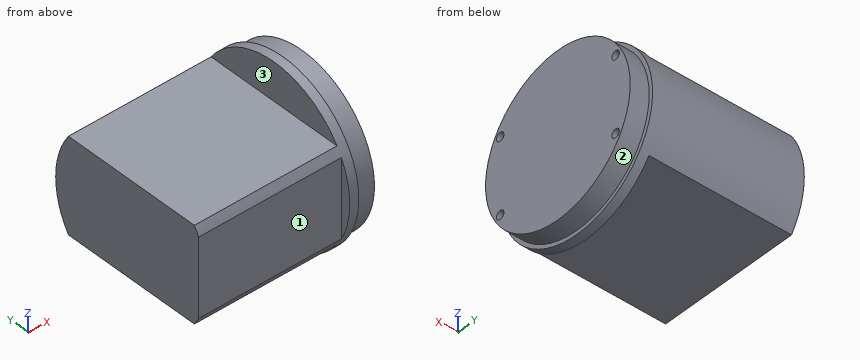
from build123d import *

# Parameters (mm, degrees)
F0_R     = 28.575
F0_R_2   = 27.2923
F1_DEPTH = 57.15
F2_DEPTH = 6.35
F4_DEPTH = 47.752
F5_R     = 1.4224
F6_DEPTH = 9.652


with BuildPart() as f1:
    # F0 (on Right) → F1 (new body)
    with BuildSketch(Plane.YZ):
        Circle(F0_R)
        Circle(F0_R_2, mode=Mode.SUBTRACT)
        Circle(F0_R_2)
    extrude(amount=-F1_DEPTH)

    # F0 (on Right) → F2 (cut)
    with BuildSketch(Plane.YZ):
        Circle(F0_R)
        Circle(F0_R_2, mode=Mode.SUBTRACT)
    extrude(amount=-F2_DEPTH, mode=Mode.SUBTRACT)

    # F3 (on face) → F4 (cut)
    with BuildSketch(Plane(origin=(-57.15, 0, 0), x_dir=(0, -1, 0), z_dir=(-1, 0, 0))):
        with BuildLine():
            ThreePointArc((-23.759524406, -15.875), (0, -28.575), (23.759524406, -15.875))
            Line((23.759524406, -15.875), (-23.759524406, -15.875))
        make_face()
        with BuildLine():
            Line((25.4, 13.0908603613), (25.4, -13.0908603613))
            ThreePointArc((25.4, -13.0908603613), (27.7699083992, -6.7351920908), (28.575, 0))
            ThreePointArc((28.575, 0), (27.7699083992, 6.7351920908), (25.4, 13.0908603613))
        make_face()
        with BuildLine():
            Line((-23.759524406, 15.875), (23.759524406, 15.875))
            ThreePointArc((23.759524406, 15.875), (0, 28.575), (-23.759524406, 15.875))
        make_face()
    extrude(amount=-F4_DEPTH, mode=Mode.SUBTRACT)

    # F5 (on face) → F6 (cut)
    with BuildSketch(Plane.YZ):
        with Locations((-21.7678, 12.573)):
            Circle(F5_R)
        with Locations((21.7678, 12.573)):
            Circle(F5_R)
        with Locations((21.7678, -12.573)):
            Circle(F5_R)
        with Locations((-21.7678, -12.573)):
            Circle(F5_R)
    extrude(amount=-F6_DEPTH, mode=Mode.SUBTRACT)


solid = f1.part
Here's how the part is built. I have some questions about the finished solid (model axes, mm). Face numbers are marked on the shaded views. A direction names the side the tool comes from. Coordinates: 2 decimals unless noted, no trailing zeros. Order: outer loops, then holes, each group sorted by start corner. A loop starts at its lowest first (then second) coordinate and runs counter-clockwise, first axis right, second up.
Item 1: For P1, Ø6, axis at x = -28.5, z = -1.5, coming from the -Y side; P2, Ø0.9, axis at y = -22.5, z = -13, coming from the +X side; P3, Ø1.5, axis at x = -32, z = 5.5, coming from the +Y side, each with a flat end and sliding along its axis, tell me the tip position at first contact or that it passes through.
Result sheet:
P1: stops at y = -25.4
P2: stops at x = -9.65
P3: stops at y = 28.18
Item 2: If we section it at A-A on z = 0: List the corners of the cut face in (x, y) for me (3 decimals).
Result sheet:
outline: (-57.15, -25.4) - (-9.398, -25.4) - (-9.398, -28.575) - (-6.35, -28.575) - (-6.35, -27.292) - (0, -27.292) - (0, 27.292) - (-6.35, 27.292) - (-6.35, 28.575) - (-57.15, 28.575) - close
Item 3: For the marked faces 1, 2 and 3, which set-ups out of +Z, -Z, +X, -X, +Y, -Y let a thin tool reach every point of the face, with its end or its side?
Result sheet:
face 1: +Z, -Z, -X, -Y
face 2: +X
face 3: +Z, -X, +Y, -Y
Item 4: If we section it at C-C on y = 0: List the corners of the cut face in (x, z) for me (3 decimals), plus the area to 3 significant figures.
Result sheet:
outline: (-57.15, -15.875) - (-9.398, -15.875) - (-9.398, -28.575) - (-6.35, -28.575) - (-6.35, -27.292) - (0, -27.292) - (0, 27.292) - (-6.35, 27.292) - (-6.35, 28.575) - (-9.398, 28.575) - (-9.398, 15.875) - (-57.15, 15.875) - close
area: 2,040 mm2
Item 5: I need wall thicknesses on line 1 (Y direction, x = -9, z = -12); line 2 (Z direction, x = -27, y = -19) (3 decimals); line 3 (X direction, y = 8.5, z = -20). Which ranges of each line are inside material? Lowest first, please.
Result sheet:
line 1: y = -25.93 to -23.07, -20.47 to 20.47, 23.07 to 25.93
line 2: z = -15.875 to 15.875
line 3: x = -9.4 to 0
Item 6: If we section it at B-B on x = -18: List the corners of the cut face in (y, z) for me (3 decimals).
Result sheet:
outline: (-25.4, -13.091) arc R28.575 ccw to (-23.76, -15.875) - (23.76, -15.875) arc R28.575 ccw to (23.76, 15.875) - (-23.76, 15.875) arc R28.575 ccw to (-25.4, 13.091) - close
Item 7: If we section it at D-D on z = 22.5: List the corners of the cut face in (x, y) for me.
Result sheet:
outline: (-9.4, -17.61) - (-6.35, -17.61) - (-6.35, -15.45) - (0, -15.45) - (0, 15.45) - (-6.35, 15.45) - (-6.35, 17.61) - (-9.4, 17.61) - close
